Autodesk Inventor part; units mm, degrees
ref_plane "Work Plane1" through (-9.3266, 85.8141, 0) normal (-1, 0, 0) x (0, 0, 1)
ref_plane "YZ Plane" through (0, 0, 0) normal (1, 0, 0) x (0, 1, 0)
ref_plane "XZ Plane" through (0, 0, 0) normal (0, 1, 0) x (-1, 0, 0)
sketch "Sketch1" plane through (0, 0, 0) normal (0, 0, 1) x (1, 0, 0)
  line L0 (-18.6531, 0) -> (18.6531, 0)
  line L1 (18.6531, 0) -> (18.6531, 35.0141)
  line L2 (18.6531, 35.0141) -> (-18.6531, 35.0141)
  line L3 (-18.6531, 35.0141) -> (-18.6531, 0)
  line L4 (0, 0) -> (0, 35.0141) construction
  line L5 (-9.3266, 35.0141) -> (-9.3266, 0) construction
  line L6 (-1.8266, 0) -> (-1.8266, 145.5582) construction
  line L7 (-16.8266, 0) -> (-16.8266, 145.5582) construction
  line L8 (-16.8266, 145.5582) -> (-1.8266, 145.5582) construction
  line L9 (-25.4, 0) -> (25.4, 0) construction
  line L10 (25.4, 0) -> (25.4, 304.8) construction
  line L11 (25.4, 304.8) -> (-25.4, 304.8) construction
  line L12 (-25.4, 304.8) -> (-25.4, 0) construction
  line L13 (-25.4, 73.1141) -> (6.7469, 73.1141)
  line L14 (6.7469, 73.1141) -> (6.7469, 174.7141)
  line L15 (6.7469, 174.7141) -> (-25.4, 174.7141)
  line L16 (-25.4, 174.7141) -> (-25.4, 73.1141)
  line L17 (-20.6375, 85.8141) -> (1.9844, 85.8141)
  line L18 (1.9844, 85.8141) -> (1.9844, 162.0141)
  line L19 (1.9844, 162.0141) -> (-20.6375, 162.0141)
  line L20 (-20.6375, 162.0141) -> (-20.6375, 85.8141)
  line L21 (-17.4625, 162.0141) -> (-17.4625, 85.8141)
  line L22 (-1.1906, 85.8141) -> (-1.1906, 162.0141)
  line L23 (-15.6766, 168.3641) -> (-2.9766, 168.3641) construction
  line L24 (-15.6766, 171.5391) -> (-2.9766, 171.5391)
  line L25 (-2.9766, 165.1891) -> (-15.6766, 165.1891)
  arc A0 (-15.6766, 171.5391) -> (-15.6766, 165.1891) centre (-15.6766, 168.3641) ccw
  arc A1 (-2.9766, 165.1891) -> (-2.9766, 171.5391) centre (-2.9766, 168.3641) ccw
  line L26 (-15.6766, 79.4641) -> (-2.9766, 79.4641) construction
  line L27 (-15.6766, 76.2891) -> (-2.9766, 76.2891)
  line L28 (-2.9766, 82.6391) -> (-15.6766, 82.6391)
  arc A2 (-15.6766, 82.6391) -> (-15.6766, 76.2891) centre (-15.6766, 79.4641) ccw
  arc A3 (-2.9766, 76.2891) -> (-2.9766, 82.6391) centre (-2.9766, 79.4641) ccw
  point P0 (0, 0)
  point P1 (-9.3266, 168.3641)
  point P2 (-9.3266, 79.4641)
  dimension "d0" = 37.3062
  dimension "d1" = 35.0141
  dimension "d2" = 15
  dimension "d3" = 50.8
  dimension "d4" = 304.8
  dimension "d5" = 101.6
  dimension "d6" = 76.2
  dimension "d7" = 4.7625
  dimension "d8" = 4.7625
  dimension "d9" = 12.7
  dimension "d10" = 12.7
  dimension "d11" = 38.1
  dimension "d12" = 3.175
  dimension "d13" = 3.175
  dimension "d14" = 12.7
  dimension "d15" = 12.7
  dimension "d16" = 3.175
  dimension "d17" = 6.35
  dimension "d18" = 3.175
  dimension "d19" = 6.35
extrude "Extrusion1" add sketch "Sketch1" along normal blind 4.7625 contours L16 L15 L14 L13 | L20 L19 L21 L17 | L21 L19 L22 L17 | L22 L19 L18 L17 | L24 A1 L25 A0 | A2 L28 A3 L27
extrude "Extrusion2" cut sketch "Sketch1" along normal blind 2.3813 contours L24 A1 L25 A0 | A2 L28 A3 L27
extrude "Extrusion3" add sketch "Sketch1" against normal blind 19.05 contours L20 L19 L21 L17 | L22 L19 L18 L17
fillet "Fillet1" radius 3.175 8 edges at (-20.6375, 85.8141, -9.525) (1.9844, 85.8141, -9.525) (-20.6375, 162.0141, -9.525) (1.9844, 162.0141, -9.525) (6.7469, 73.1141, 2.3813) (-25.4, 73.1141, 2.3813) (-25.4, 174.7141, 2.3813) (6.7469, 174.7141, 2.3813)
ref_plane "Work Plane1" through (-9.3266, 85.8141, 0) normal (-1, 0, 0) x (0, 0, 1)
sketch "Sketch2" plane through (0, 0, -19.05) normal (0, 0, -1) x (-1, 0, 0)
  arc A0 (20.6375, 158.8391) -> (17.4625, 162.0141) centre (17.4625, 158.8391) ccw
  line L0 (17.4625, 162.0141) -> (17.4625, 85.8141)
  arc A1 (17.4625, 85.8141) -> (20.6375, 88.9891) centre (17.4625, 88.9891) ccw
  line L1 (20.6375, 88.9891) -> (20.6375, 158.8391)
  arc A2 (20.5105, 158.8391) -> (17.5895, 161.8844) centre (17.4625, 158.8391) ccw
  line L2 (20.5105, 158.8391) -> (20.5105, 88.9891)
  arc A3 (17.5895, 85.9437) -> (20.5105, 88.9891) centre (17.4625, 88.9891) ccw
  line L3 (17.5895, 85.9437) -> (17.5895, 161.8844)
  point P0 (0, 0)
  dimension "d27" = 0.127
extrude "Extrusion4" cut sketch "Sketch2" against normal up to surface (19.05 mm away)
mirror "Mirror1" about plane through (-9.3266, 85.8141, 0) normal (-1, 0, 0) of "Extrusion4"
equation "\"d9\" = d10"
properties part number "Maglock Aligner" material "Polyethylene, High Density"
Input: part model. Units: mm. Frame: model coordinates. A direction names the side the tool comes from. Give positions to 0.01 mm unless a question says otherwise; leave off trailing zeros. Order: outer loops, then holes, each group sorted by start corner. A loop starts at its lowest first (then second) coordinate and runs counter-clockwise, first axis right, second up. Notation, with made-up numbers: M 78.25,-14.5 L 137.25,-14.5 A13 cw 137.25,-7.5 Z; hole C 35.5,41 d7. An arc over 180 degrees is marked long. Return JSON: item names as keys, results as strings.
Item 1: Pull-direction query (X, two-part tool) for faces 6 (the cylindrical face through (5.8, 173.8, 2.4)), 7 (the cylindrical face through (-24.445, 173.809, 2.415)), 8 (the flat face through (-9, 82.639, 1)); classes: +X half, -X half, draft (parallel to the pull), parting line (faces both ways), or undercut.
Solutions:
{"face 6": "+X half", "face 7": "-X half", "face 8": "undercut"}
Item 2: First-contact query: P1, Ø5, axis at x = -13, z = -5.5, coming from the +Y side; P2, Ø4, axis at y = 109.5, z = -5, coming from the -X side; P3, Ø7, axis at x = -11.5, y = 79.5, coming from the -Z side; P4, Ø8, axis at x = -22, z = -13, coming from the +Y side. Flat tips, straight axial feed; report the tip coordinate or a pass-through.
Solutions:
{"P1": "through", "P2": "x = -20.51", "P3": "z = 0", "P4": "y = 161.84"}
Item 3: Cut plane C-C (y = 146). Return loops of the section in (x, z).
Solutions:
{"outline": "M -25.4,0 L -20.51,0 L -20.51,-19.05 L -17.59,-19.05 L -17.59,0 L -1.06,0 L -1.06,-19.05 L 1.86,-19.05 L 1.86,0 L 6.75,0 L 6.75,4.76 L -25.4,4.76 Z"}
Item 4: Ray query, probe 1 along X at (y, z) = (114, -10.75); probe 2 along Z at (x, y) = (-17.5, 119); probe 3 along Z at (x, y) = (-6.5, 165.5). Return the intervals inside material, ascending.
Solutions:
{"probe 1": "-20.51 to -17.59, -1.06 to 1.86", "probe 2": "0 to 4.76", "probe 3": "2.38 to 4.76"}
Item 5: Access query for faces 1 (the flat face through (-9, 165.189, 1)), 2 (the flat face through (-17.59, 123, -10)), 3 (the flat face through (1.857, 123, -10)), 4 (the flat face through (-20.51, 124, -10)), 5 (the cylindrical face through (1.03, 86.9, -9.66)). Directions: +Z, -Z, +X, -X, +Y, -Y. A direction counts if a zero-diameter tool reaches every point of the face in a straight line with its end or side. Return the directions, or none.
Solutions:
{"face 1": "-Z", "face 2": "-Z, +Y, -Y", "face 3": "-Z, +X, +Y, -Y", "face 4": "-Z, -X, +Y, -Y", "face 5": "-Z, +X, -Y"}
Item 6: Cut plane A-A (z = 1). Return loops of the section in (x, y) (3 decimals), then the cut area to 3 significant figures.
Solutions:
{"outline": "M -25.4,76.289 A3.175 ccw -22.225,73.114 L 3.572,73.114 A3.175 ccw 6.747,76.289 L 6.747,171.539 A3.175 ccw 3.572,174.714 L -22.225,174.714 A3.175 ccw -25.4,171.539 Z; hole M -15.677,76.289 L -2.977,76.289 A3.175 ccw -2.977,82.639 L -15.677,82.639 A3.175 ccw Z; hole M -15.677,165.189 L -2.977,165.189 A3.175 ccw -2.977,171.539 L -15.677,171.539 A3.175 ccw Z", "area": "3,030 mm^2"}
Item 7: Cut plane B-B (x = -4.5). Return loops of the section in (y, z).
Solutions:
{"outline": "M 73.11,0 L 76.29,0 L 76.29,2.38 L 82.64,2.38 L 82.64,0 L 165.19,0 L 165.19,2.38 L 171.54,2.38 L 171.54,0 L 174.71,0 L 174.71,4.76 L 73.11,4.76 Z"}
Item 8: Cut plane D-D (z = -6). Return loops of the section in (x, y).
Solutions:
{"outline": "M -20.51,88.99 A3.05 ccw -17.59,85.94 L -17.59,161.88 A3.05 ccw -20.51,158.84 Z; M -1.06,85.94 A3.05 ccw 1.86,88.99 L 1.86,158.84 A3.05 ccw -1.06,161.88 Z"}
